Could you check a few things on this model? Use its own coordinates, in mm. A direction names the side the tool comes from. Give positions to 0.01 mm unless a question says otherwise; leave off trailing zeros. Order: outer loops, then holes, each group sorted by start corner. A loop starts at its lowest first (then second) coordinate and runs counter-clockwise, first axis right, second up. Notation, with made-up numbers: (-37.75, -20.75) -> (-1.75, -20.75) arc R33 ccw to (-1.75, 7.25) -> close; hole circle Ø9 at (-4.75, -17.5). An arc over 180 degrees is marked (long way). Write each question's results on one line, items separated by ' | '.
```python
from build123d import *

# Parameters (mm, degrees)
SKETCH_1_R       = 1.5
M3X8_DEPTH       = 8
EXTRUDE_START    = 8
EXTRUDE_D9_DEPTH = 3


with BuildPart() as part:
    # 草图1 → M3x8简化螺杆 (new body)
    with BuildSketch(Plane.XY):
        Circle(SKETCH_1_R)
    extrude(amount=M3X8_DEPTH)

    # 草图2 → D9十二边手拧头 (add)
    with BuildSketch(Plane.XY.offset(EXTRUDE_START)):
        Polygon((4.5, 0), (3.897114317, 2.25), (2.25, 3.897114317), (0, 4.5), (-2.25, 3.897114317), (-3.897114317, 2.25), (-4.5, 0), (-3.897114317, -2.25), (-2.25, -3.897114317), (0, -4.5), (2.25, -3.897114317), (3.897114317, -2.25), align=None)
    extrude(amount=EXTRUDE_D9_DEPTH)


solid = part.part
```
Q1. Suppose I cut it at C-C on x = -0.5. Please give me the cut outline in (y, z).
Here are the results:
outline: (-4.37, 8) -> (-1.41, 8) -> (-1.41, 0) -> (1.41, 0) -> (1.41, 8) -> (4.37, 8) -> (4.37, 11) -> (-4.37, 11) -> close
Q2. I need wall thicknesses on line 1 along Z through (x, y) = (2.25, -0.25); line 2 along Y through (x, z) = (-0.75, 3.75); line 3 along X through (y, z) = (3, 8.25). Which ranges of each line are inside material? Lowest first, please.
Here are the results:
line 1: z = 8 to 11 | line 2: y = -1.3 to 1.3 | line 3: x = -3.15 to 3.15
Q3. Suppose I cut it at B-B on z = 10. Please give me the cut outline in (x, y).
Here are the results:
outline: (-4.5, 0) -> (-3.9, -2.25) -> (-2.25, -3.9) -> (0, -4.5) -> (2.25, -3.9) -> (3.9, -2.25) -> (4.5, 0) -> (3.9, 2.25) -> (2.25, 3.9) -> (0, 4.5) -> (-2.25, 3.9) -> (-3.9, 2.25) -> close
Q4. Suppose I cut it at A-A on y = 0.75. Please give me the cut outline in (x, z).
Here are the results:
outline: (-4.3, 8) -> (-1.3, 8) -> (-1.3, 0) -> (1.3, 0) -> (1.3, 8) -> (4.3, 8) -> (4.3, 11) -> (-4.3, 11) -> close
Q5. I'm going to push a flat-ended pin straight in: pin 1 Ø4 at (y, z) = (2.5, 2) entering from +X. Where does the tip first touch, or does it pass through?
Here are the results:
pin 1: stops at x = 1.41
Q6. Suppose I cut it at D-D on z = 5. Please give me the cut outline in (x, y), and give its area (3 significant figures).
Here are the results:
outline: circle Ø3 at (0, 0) | area: 7.07 mm²
Q7. For faces 1 (the cylindrical face through (-1.5, 0.07, 3.94)), 2 (the flat face through (-1.109, 4.203, 9.479)), which set-ups out of +Z, -Z, +X, -X, +Y, -Y let a thin tool reach every point of the face, with its end or its side?
Here are the results:
face 1: -Z | face 2: +Z, -Z, -X, +Y
